Part model, mm, in its own coordinate system. Face numbers are marked on the shaded views. Give positions to 0.01 mm unless a question says otherwise; leave off trailing zeros. Write each loop counter-clockwise with the first axis right and the second up, starting at its lowest first coordinate (ties: lowest second). Pieces come first, ordered by that corner, then holes. Notation, with made-up numbers: M 79,-27 L 134,-27 A17 cw 134,-18 Z; hole C 84.5,23.5 d8. An arc over 180 degrees is marked long. Write item = value, one per line. Start each with the question number.
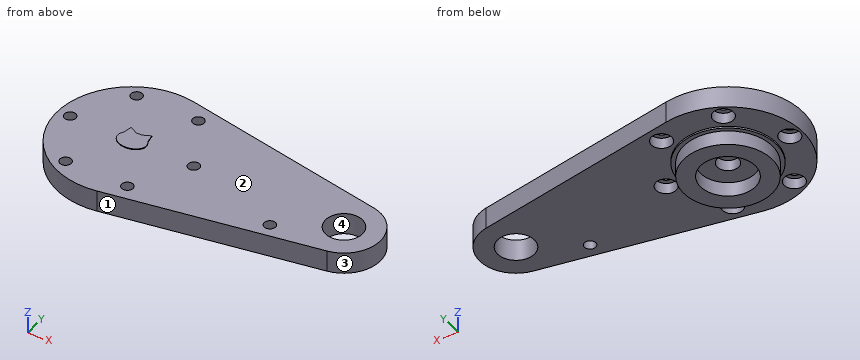
from build123d import *

# Parameters (mm, degrees)
SKETCH_1_R          = 5.15
EXTRUDE_1_DEPTH     = 6
SKETCH_3_R          = 1.6
CUT_EXTRUDE_2_DEPTH = 74.471235868
SKETCH_5_R          = 13.5
EXTRUDE_3_DEPTH     = 0.5
SKETCH_4_R          = 12.35
SKETCH_4_R_2        = 7.65
EXTRUDE_2_DEPTH     = 4
SKETCH_6_R          = 3
CUT_EXTRUDE_3_DEPTH = 3
SKETCH_7_R          = 2.85
CUT_EXTRUDE_4_DEPTH = 3
EXTRUDE_4_DEPTH     = 0.2
SKETCH_10_R         = 1.6
CUT_EXTRUDE_6_DEPTH = 74.487839262


with BuildPart() as part:
    # 草图1 → 凸台-拉伸1 (new body)
    with BuildSketch(Plane.XY):
        with BuildLine():
            Line((61.835458333, -9.98266461), (3.7975, -20.653788847))
            ThreePointArc((3.7975, -20.653788847), (-21, 0), (3.7975, 20.653788847))
            Line((3.7975, 20.653788847), (61.835458333, 9.98266461))
            ThreePointArc((61.835458333, 9.98266461), (70.15, 0), (61.835458333, -9.98266461))
        make_face()
        with Locations((60, 0)):
            Circle(SKETCH_1_R, mode=Mode.SUBTRACT)
    extrude(amount=EXTRUDE_1_DEPTH)

    # 草图3 → 切除-拉伸2 (cut, through all)
    with BuildSketch(Plane.XY.offset(6)):
        with Locations((8.75, 15.155444566)):
            Circle(SKETCH_3_R)
        with Locations((17.5, 0)):
            Circle(SKETCH_3_R)
        with Locations((8.75, -15.155444566)):
            Circle(SKETCH_3_R)
        with Locations((-8.75, -15.155444566)):
            Circle(SKETCH_3_R)
        with Locations((-17.5, 0)):
            Circle(SKETCH_3_R)
        with Locations((-8.75, 15.155444566)):
            Circle(SKETCH_3_R)
    extrude(amount=-CUT_EXTRUDE_2_DEPTH, mode=Mode.SUBTRACT)

    # 草图5 → 凸台-拉伸3 (add)
    with BuildSketch(Plane(origin=(0, 0, 0), x_dir=(-1, 0, 0), z_dir=(0, 0, -1))):
        with Locations(Location((0, 0, 0), (0, 0, 180))):
            Circle(SKETCH_5_R)
    extrude(amount=EXTRUDE_3_DEPTH)

    # 草图4 → 凸台-拉伸2 (add)
    with BuildSketch(Plane(origin=(0, 0, -0.5), x_dir=(-1, 0, 0), z_dir=(0, 0, -1))):
        Circle(SKETCH_4_R)
        Circle(SKETCH_4_R_2, mode=Mode.SUBTRACT)
    extrude(amount=EXTRUDE_2_DEPTH)

    # 草图6 → 切除-拉伸3 (cut)
    with BuildSketch(Plane(origin=(0, 0, -0.5), x_dir=(-1, 0, 0), z_dir=(0, 0, -1))):
        Circle(SKETCH_6_R)
    extrude(amount=-CUT_EXTRUDE_3_DEPTH, mode=Mode.SUBTRACT)

    # 草图7 → 切除-拉伸4 (cut)
    with BuildSketch(Plane(origin=(0, 0, 0), x_dir=(-1, 0, 0), z_dir=(0, 0, -1))):
        with Locations((8.75, 15.155444566)):
            Circle(SKETCH_7_R)
        with Locations((17.5, 0)):
            Circle(SKETCH_7_R)
        with Locations((8.75, -15.155444566)):
            Circle(SKETCH_7_R)
        with Locations((-8.75, -15.155444566)):
            Circle(SKETCH_7_R)
        with Locations((-17.5, 0)):
            Circle(SKETCH_7_R)
        with Locations((-8.75, 15.155444566)):
            Circle(SKETCH_7_R)
    extrude(amount=-CUT_EXTRUDE_4_DEPTH, mode=Mode.SUBTRACT)

    # 草图9 → 凸台-拉伸4 (add)
    with BuildSketch(Plane.XY.offset(6)):
        with BuildLine():
            Line((-2.954769624, 4.033526555), (-3.40491347, 1.574386356))
            add(Edge.make_bspline(
                [(-3.40491347, 1.574386356), (-7.165153372, -3), (0, -3), (7.165153372, -3), (3.40491347, 1.574386356)],
                knots=[2.589117856, 2.589117856, 2.589117856, 4.71238898, 4.71238898, 6.835660105, 6.835660105, 6.835660105], degree=2, weights=[1, 0.487444637, 1, 0.487444637, 1]))
            Line((3.40491347, 1.574386356), (2.954769624, 4.033526555))
            Line((2.954769624, 4.033526555), (0.7, 2.9537053))
            add(Edge.make_bspline(
                [(0.7, 2.9537053), (0, 3.047020297), (-0.7, 2.9537053)],
                knots=[1.394890559, 1.394890559, 1.394890559, 1.746702095, 1.746702095, 1.746702095], degree=2, weights=[1, 0.984568433, 1]))
            Line((-0.7, 2.9537053), (-2.954769624, 4.033526555))
        make_face()
    extrude(amount=EXTRUDE_4_DEPTH)

    # 草图10 → 切除-拉伸6 (cut, through all)
    with BuildSketch(Plane(origin=(0, 0, 0), x_dir=(-1, 0, 0), z_dir=(0, 0, -1))):
        with Locations((-45, -9)):
            Circle(SKETCH_10_R)
    extrude(amount=-CUT_EXTRUDE_6_DEPTH, mode=Mode.SUBTRACT)


solid = part.part
Q1. Probe line 1 along Y through (x, z) = (-8.75, 5.25); line 2 along Z through (x, y) = (42.5, 3); line 3 along Y through (x, z) = (8.75, 4.9). List the from-to ranges inside material, lowest first.
Q2. Drop flat-ended pins along their axis: P1, Ø4.5, axis at x = 9, y = -16, coming from the -Z side; P2, Ø1, axis at x = 0, y = 9.5, coming from the +Z side; P3, Ø3, axis at x = -10, y = -15.5, coming from the -Z side; P4, Ø8, axis at x = 60, y = 0, coming from the +Z side. Give the stop position or say it passes through.
Q3. Slice it at D-D (z = -1.5). Give the cut face in (x, y), and give its area (3 significant figures).
Q4. Two-plate mould, pull along Y, no slides. Class the marked faces 1, 2, 3 and 4: +Y half, -Y half, draft (parallel to the pull), parting line (faces both ways), or undercut.
Q5. Slice it at A-A (x = 17.5). Give the cut face in (y, z), and give its area (3 significant figures).
Q6. Slice it at C-C (y = 6). Give the cut face in (x, z), and give its area (3 significant figures).
Q7. Slice it at B-B (x = -8.75). Give the cut face in (y, z).
Working result:
q1.line_1 = -19.09 to -16.76, -13.56 to 13.56, 16.76 to 19.09
q1.line_2 = 0 to 6
q1.line_3 = -19.74 to -16.76, -13.56 to 13.56, 16.76 to 19.74
q2.P1 = 0
q2.P2 = 6
q2.P3 = 3
q2.P4 = through
q3.outline = C 0,0 d24.7; hole C 0,0 d15.3
q3.area = 295 mm2
q4.face_1 = -Y half
q4.face_2 = draft
q4.face_3 = parting line
q4.face_4 = undercut
q5.outline = M -18.13,0 L -2.85,0 L -2.85,3 L -1.6,3 L -1.6,6 L -18.13,6 Z; M 1.6,3 L 2.85,3 L 2.85,0 L 18.13,0 L 18.13,6 L 1.6,6 Z
q5.area = 191 mm2
q6.outline = M -20.12,0 L -12.09,0 L -12.09,-0.5 L -10.79,-0.5 L -10.79,-4.5 L -4.75,-4.5 L -4.75,-0.5 L 4.75,-0.5 L 4.75,-4.5 L 10.79,-4.5 L 10.79,-0.5 L 12.09,-0.5 L 12.09,0 L 68.19,0 L 68.19,6 L -20.12,6 Z
q6.area = 590 mm2
q7.outline = M -19.09,0 L -18.01,0 L -18.01,3 L -16.76,3 L -16.76,6 L -19.09,6 Z; M -13.56,3 L -12.31,3 L -12.31,0 L -10.28,0 L -10.28,-0.5 L -8.72,-0.5 L -8.72,-4.5 L 8.72,-4.5 L 8.72,-0.5 L 10.28,-0.5 L 10.28,0 L 12.31,0 L 12.31,3 L 13.56,3 L 13.56,6 L -13.56,6 Z; M 16.76,3 L 18.01,3 L 18.01,0 L 19.09,0 L 19.09,6 L 16.76,6 Z
